```python
from build123d import *

# Parameters (mm, degrees)
F0_W     = 6.5
F0_H     = 6.5
F1_DEPTH = 4.6
F2_R     = 3
F3_DEPTH = 14.4


with BuildPart() as f1:
    # F0 (on Top) → F1 (new body)
    with BuildSketch(Plane.XY):
        Rectangle(F0_W, F0_H)
    extrude(amount=F1_DEPTH)

    # F2 (on face) → F3 (join)
    with BuildSketch(Plane.XY.offset(4.6)):
        Circle(F2_R)
    extrude(amount=F3_DEPTH)

    # F4 (on Right) → F5 (revolve)
    with BuildSketch(Plane.YZ):
        with BuildLine():
            ThreePointArc((0, -3.8), (4.552901, -2.80459), (8.275, 0))
            Line((8.275, 0), (0, 0))
            Line((0, 0), (0, -3.8))
        make_face()
    revolve(axis=Axis((0, 0, -1.9), (0, 0, -1)))


solid = f1.part
```
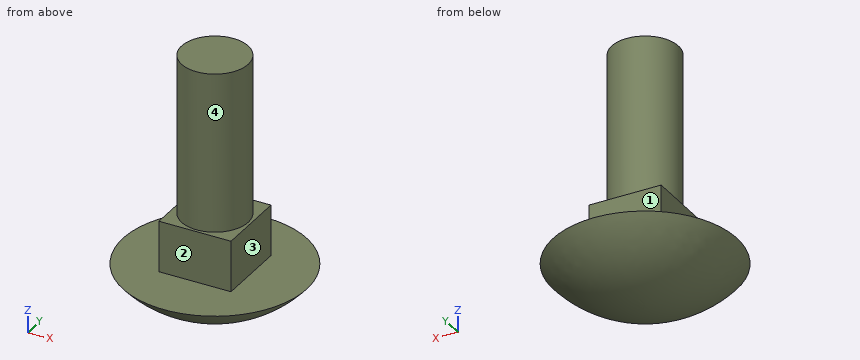
Geometry check sheet. Reference: the model listing, model coordinates, mm. Face numbers are marked on the shaded views. A direction names the side the tool comes from. Give positions to 0.01 mm unless a question says otherwise; leave off trailing zeros. Order: outer loops, then holes, each group sorted by start corner. A loop starts at its lowest first (then second) coordinate and runs counter-clockwise, first axis right, second up. Notation, with made-up numbers: (11, 22) - (31, 22) arc R13 cw to (31, 46) - close; hole circle Ø1 at (64.5, 83). An arc over 180 degrees is marked (long way). Answer in a Markdown table with one row per item. Add a question column.
Q1. Material ranges on probe 1 along Y at (x, z) = (1.25, 3); probe 2 along Z at (x, y) = (0.75, 4.5); probe 3 along Y at (x, z) = (6.5, -1), recorded low to high. Write a range as from..to.
Q2. Cross-section at A-A, the plane z = 3.75. Enter the section's corners in (x, y).
Q3. Cross-section at B-B, the plane z = 13.5. Enter the section's corners in (x, y), then the cut area to 3 significant figures.
Q4. Tool access check on the marked faces 1, 2, 3 and 4. Record the directions out of +Z, -Z, +X, -X, +Y, -Y that give a thin tool (end or side, any length) a straight path to the whole face; none if there is none.
Q5. Gauge pin test, flat ends, axial feed: pin 1 (1 mm diameter, centred on x = 1, y = 3, fed in from -Z); pin 2 (3.5 mm diameter, centred on y = -1, z = 3.5, fed in from -X); pin 3 (2.5 mm diameter, centred on x = 1, z = 2.5, fed in from -Y); pin 4 (8.5 mm diameter, centred on x = -3, y = 4, fed in from +Z). Record the tip position at first contact, or that the pin passes through.
Check values:
| question | item | result |
|---|---|---|
| 1 | probe 1 | y = -3.25..3.25 |
| 1 | probe 2 | z = -2.8..0 |
| 1 | probe 3 | y = -3.32..3.32 |
| 2 | outline | (-3.25, -3.25) - (3.25, -3.25) - (3.25, 3.25) - (-3.25, 3.25) - close |
| 3 | outline | circle Ø6 at (0, 0) |
| 3 | area | 28.3 mm^2 |
| 4 | face 1 | +Z, +X, -X, +Y |
| 4 | face 2 | +Z, +X, -X, -Y |
| 4 | face 3 | +Z, +X, +Y, -Y |
| 4 | face 4 | +Z |
| 5 | pin 1 | stops at z = -3.47 |
| 5 | pin 2 | stops at x = -3.25 |
| 5 | pin 3 | stops at y = -3.25 |
| 5 | pin 4 | stops at z = 19 |
